Geometry check sheet. Reference: drawing and pictorial views, mm from the part's lowest x, y, z. Round coordinates to 2 decimals unless told otherwise and drop trailing zeros. Loops run counter-clockwise (first coordinate to the right, second up) from the corner with the lowest first, then second, coordinate; pieces in that order, holes last. Notation, with made-up numbers: (-9, 86) -> (9, 86) arc R19 cw to (9, 119) -> close; hole circle Ø2 at (7, 2). An arc over 180 degrees is marked (long way). Write item = value, one per line.
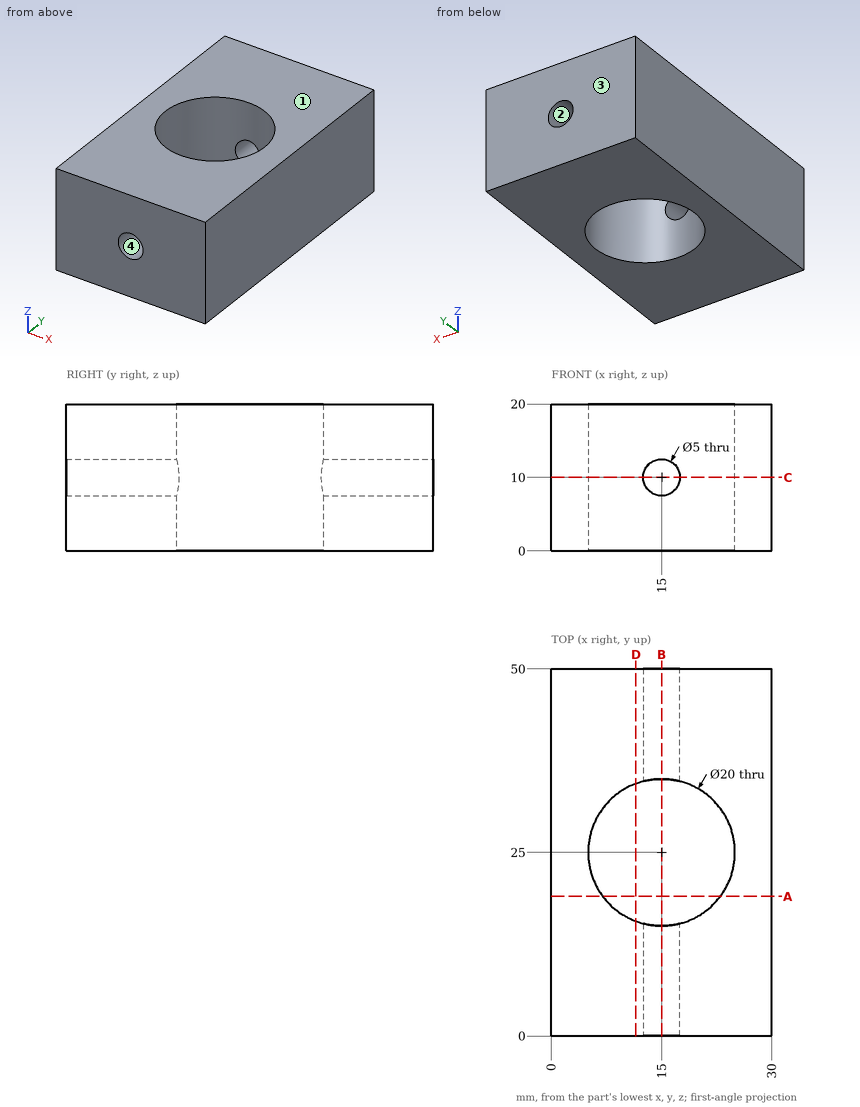
(1) Sectioned sample at A-A, the plane y = 19. Record the cut outline in (x, z), and give its area (3 significant figures).
Filled sheet:
outline = (0, 0) -> (7, 0) -> (7, 20) -> (0, 20) -> close; (23, 0) -> (30, 0) -> (30, 20) -> (23, 20) -> close
area = 280 mm2
(2) Material ranges on probe 1 along Z at (x, y) = (15, 38.75); probe 2 along X at (y, z) = (18.5, 18.75); probe 3 along Y at (x, z) = (15, 7.25), recorded low to high. Write a range as from..to.
Filled sheet:
probe_1 = 0..7.5, 12.5..20
probe_2 = 0..7.4, 22.6..30
probe_3 = 0..15, 35..50
(3) Go/stop test with a flat-tipped pin: pin 1 Ø16 at (x, y) = (15, 25) entering from -Z. Record where the tip stops, or that it passes through.
Filled sheet:
pin_1 = through
(4) Sectioned sample at B-B, the plane x = 15. Record the cut outline in (y, z).
Filled sheet:
outline = (0, 0) -> (15, 0) -> (15, 7.5) -> (0, 7.5) -> close; (0, 12.5) -> (15, 12.5) -> (15, 20) -> (0, 20) -> close; (35, 0) -> (50, 0) -> (50, 7.5) -> (35, 7.5) -> close; (35, 12.5) -> (50, 12.5) -> (50, 20) -> (35, 20) -> close
(5) Draft check along Z on the marked faces 1, 2, 3 and 4. Enter one of: released by +Z, released by -Z, zero draft, split by the parting line, or undercut.
Filled sheet:
face_1 = released by +Z
face_2 = undercut
face_3 = zero draft
face_4 = undercut
(6) Sectioned sample at D-D, the plane x = 11.5. Record the cut outline in (y, z).
Filled sheet:
outline = (0, 0) -> (15.63, 0) -> (15.63, 20) -> (0, 20) -> close; (34.37, 0) -> (50, 0) -> (50, 20) -> (34.37, 20) -> close
(7) Sectioned sample at C-C, the plane z = 10. Record the cut outline in (x, y).
Filled sheet:
outline = (0, 0) -> (12.5, 0) -> (12.5, 15.32) arc R10 cw to (12.5, 34.68) -> (12.5, 50) -> (0, 50) -> close; (17.5, 0) -> (30, 0) -> (30, 50) -> (17.5, 50) -> (17.5, 34.68) arc R10 cw to (17.5, 15.32) -> close
